from build123d import *

# Parameters (mm, degrees)
SKETCH1_W           = 30
SKETCH1_H           = 30
SKETCH1_R           = 1
BOSS_EXTRUDE2_DEPTH = 1
SKETCH2_W           = 15
SKETCH2_H           = 13
BOSS_EXTRUDE3_DEPTH = 2.8
BOSS_EXTRUDE4_DEPTH = 4


with BuildPart() as part:
    # Sketch1 → Boss-Extrude2 (new body)
    with BuildSketch(Plane(origin=(0, 0, 0), x_dir=(1, 0, 0), z_dir=(0, 1, 0))):
        with Locations((2.382352941, -5.426470588)):
            Rectangle(SKETCH1_W, SKETCH1_H)
        with Locations(Location((-10.617647059, 7.573529412, 0), (0, 0, 270))):  # turned: the seam where the file's is
            Circle(SKETCH1_R, mode=Mode.SUBTRACT)
        with Locations(Location((15.382352941, 7.573529412, 0), (0, 0, 270))):  # turned: the seam where the file's is
            Circle(SKETCH1_R, mode=Mode.SUBTRACT)
        with Locations(Location((15.382352941, -18.426470588, 0), (0, 0, 270))):  # turned: the seam where the file's is
            Circle(SKETCH1_R, mode=Mode.SUBTRACT)
        with Locations(Location((-10.617647059, -18.426470588, 0), (0, 0, 270))):  # turned: the seam where the file's is
            Circle(SKETCH1_R, mode=Mode.SUBTRACT)
    extrude(amount=BOSS_EXTRUDE2_DEPTH)

    # Sketch2 → Boss-Extrude3 (add)
    with BuildSketch(Plane(origin=(0, 1, 0), x_dir=(1, 0, 0), z_dir=(0, 1, 0))):
        with Locations((5.882352941, -10.926470588)):
            Rectangle(SKETCH2_W, SKETCH2_H)
    extrude(amount=BOSS_EXTRUDE3_DEPTH)

    # Sketch3 → Boss-Extrude4 (add)
    with BuildSketch(Plane.XZ):
        with BuildLine():
            Line((-5.926151738, 17.926470588), (10.69085762, 17.926470588))
            ThreePointArc((10.69085762, 17.926470588), (13.654692385, 16.698810032), (14.882352941, 13.734975267))
            Line((14.882352941, 13.734975267), (14.882352941, -2.882034091))
            ThreePointArc((14.882352941, -2.882034091), (13.654692385, -5.845868856), (10.69085762, -7.073529412))
            Line((10.69085762, -7.073529412), (-5.926151738, -7.073529412))
            ThreePointArc((-5.926151738, -7.073529412), (-8.889986503, -5.845868856), (-10.117647059, -2.882034091))
            Line((-10.117647059, -2.882034091), (-10.117647059, 13.734975267))
            ThreePointArc((-10.117647059, 13.734975267), (-8.889986503, 16.698810032), (-5.926151738, 17.926470588))
        make_face()
    extrude(amount=BOSS_EXTRUDE4_DEPTH)


solid = part.part
Check sheet for the modelled part. Datum: model origin and axes. Units: mm. A direction names the side the tool comes from. Round coordinates to 2 decimals unless told otherwise and drop trailing zeros. Loops run counter-clockwise (first coordinate to the right, second up) from the corner with the lowest first, then second, coordinate; pieces in that order, holes last. Notation, with made-up numbers: (84, 22.5) - (140, 22.5) arc R12 ccw to (140, 44.5) - close; hole circle Ø1 at (34, 19.5). An arc over 180 degrees is marked (long way). Answer as CSV lines item,"result". Start each with the question number.
Item 1: Release check for a two-part mould opening along Z. For faces 1 (the cylindrical face through (15.426, 0.493, 17.427)), 2 (the cylindrical face through (-8.857, -1.972, -5.878)), 3 (the flat face through (3, -4, 6)), 4 (the flat face through (2.2, 0.5, 20.426)) record: +Z half, -Z half, draft (parallel to the pull), parting line (faces both ways), or undercut.
Item 2: Set-up check for faces 5 (the flat face through (-11, 0, 4)), 6 (the flat face through (-1.618, 2, 11)), 7 (the cylindrical face through (13.622, -1.972, 16.731)), 8 (the flat face through (6, 2, 17.426)), 9 (the flat face through (6, 2, 4.426)): record each of +Z, -Z, +X, -X, +Y, -Y from which the full face is reachable in a straight line by a thin tool's end or side.
Item 3: Section check C-C (y = -0.5). Record the boundary of the cut face in (x, z).
Item 4: Section check A-A (z = 3.25). Record the boundary of the cut face in (x, y), and give its area (3 significant figures).
Item 5: Scan lines: line 1 (X direction, y = -0.25, z = 9.5); line 2 (X direction, y = 2.25, z = 16.75); line 3 (Y direction, x = -2.75, z = 13.25). Record each from-to range of solid material in increasing order. Write a range as [from, to].
Item 6: Section check D-D (x = -1). Record the boundary of the cut face in (y, z).
Item 7: Depth check by flat-ended pin: P1, Ø2, axis at x = 2.5, y = -1.5, coming from the -Z side; P2, Ø2.5, axis at x = -10.62, z = -7.57, coming from the -Y side; P3, Ø0.8, axis at y = 2.5, z = 13.5, coming from the -X side. Enter the tip coordinate at first touch or a pass-through.
Item 8: Section check B-B (x = 15.75). Record the boundary of the cut face in (y, z).
Report:
1,face 1,"undercut"
1,face 2,"-Z half"
1,face 3,"draft"
1,face 4,"+Z half"
2,face 5,"-Y"
2,face 6,"+Z, -Z, -X, +Y"
2,face 7,"+Z, +X, -Y"
2,face 8,"+Z, +X, -X, +Y"
2,face 9,"-Z, +X, -X, +Y"
3,outline,"(-10.12, -2.88) arc R4.19 ccw to (-5.93, -7.07) - (10.69, -7.07) arc R4.19 ccw to (14.88, -2.88) - (14.88, 13.73) arc R4.19 ccw to (10.69, 17.93) - (-5.93, 17.93) arc R4.19 ccw to (-10.12, 13.73) - close"
4,outline,"(-12.62, 0) - (-10.12, 0) - (-10.12, -4) - (14.88, -4) - (14.88, 0) - (17.38, 0) - (17.38, 1) - (-12.62, 1) - close"
4,area,"130 mm2"
5,line 1,"x = [-10.12, 14.88]"
5,line 2,"x = [-1.62, 13.38]"
5,line 3,"y = [-4, 1]"
6,outline,"(-4, -7.07) - (0, -7.07) - (0, -9.57) - (1, -9.57) - (1, 4.43) - (3.8, 4.43) - (3.8, 17.43) - (1, 17.43) - (1, 20.43) - (0, 20.43) - (0, 17.93) - (-4, 17.93) - close"
7,P1,"stops at z = -7.07"
7,P2,"stops at y = 0"
7,P3,"stops at x = -1.62"
8,outline,"(0, -9.57) - (1, -9.57) - (1, -8.5) - (0, -8.5) - close; (0, -6.64) - (1, -6.64) - (1, 17.5) - (0, 17.5) - close; (0, 19.36) - (1, 19.36) - (1, 20.43) - (0, 20.43) - close"
